Autodesk Inventor part; units mm, degrees
ref_plane "YZ Plane" through (0, 0, 0) normal (1, 0, 0) x (0, 1, 0)
ref_plane "XZ Plane" through (0, 0, 0) normal (0, 1, 0) x (-1, 0, 0)
ref_plane "XY Plane" through (0, 0, 0) normal (0, 0, 1) x (1, 0, 0)
sketch "Szkic1" plane through (0, 0, 0) normal (1, 0, 0) x (0, 1, 0)
  line L0 (-11.2, 0) -> (11.2, 0)
  line L1 (0, -11.2) -> (0, 11.2)
  circle A0 centre (0, 0) radius 8
  dimension "d0" = 16
extrude "Wyciągnięcie proste1" add sketch "Szkic1" along normal blind 212
sketch "Szkic2" plane through (212, 0, 0) normal (1, 0, 0) x (0, 0, -1)
  circle A0 centre (0, 0) radius 8
  line L0 (0, -11.2) -> (0, 11.2)
  line L1 (16, 0) -> (-12, 0)
  circle A1 centre (-4, 0) radius 1
  circle A2 centre (4, 0) radius 1
  point P0 (12, 0)
  dimension "d11" = 10
  dimension "d4" = 16
  dimension "d5" = 2
  dimension "d8" = 8
extrude "Wyciągnięcie proste2" add sketch "Szkic2" along normal blind 7 contours A2 L1 | L1 A2 | A1 L1 | L1 A1
sketch "Szkic3" plane through (0, 0, 0) normal (-1, 0, 0) x (0, 0, 1)
  circle A0 centre (0, 0) radius 8
  line L0 (-11.2, 0) -> (11.2, 0)
  line L1 (0, -11.2) -> (0, 11.2)
  circle A1 centre (-4, 0) radius 1
  circle A2 centre (4, 0) radius 1
  dimension "d19" = 10
  dimension "d15" = 2
  dimension "d16" = 16
  dimension "d22" = 8
extrude "Wyciągnięcie proste3" add sketch "Szkic3" along normal blind 7 contours A2 L0 | L0 A2 | A1 L0 | L0 A1
equation "\"d8\" = 0.5 * d4"
equation "\"d22\" = 0.5 * d16"
properties part number "świetlówka"
Could you check a few things on this model? Use its own coordinates, in mm. Coordinates: 2 decimals unless noted, no trailing zeros. Loops run counter-clockwise (first coordinate to the right, second up) from the corner with the lowest first, then second, coordinate; pieces in that order, holes last. Notation, with made-up numbers: M -37,-27 L -16,-27 A12 ccw -16,-16 Z; hole C 55,-20.75 d11. An arc over 180 degrees is marked long. Put each result on its own line as item: value. Start each with the question number.
(1) Suppose I cut it at B-B on y = -4. Please give me the cut outline in (x, z), then the cut area to 3 significant figures.
(2) I need wall thicknesses on line 1 (X direction, y = 4.75, z = 0); line 2 (Y direction, x = 120, z = 0.25); line 3 (Y direction, x = 32, z = -6.25). Which ranges of each line are inside material? Lowest first, please. Write a range as from..to.
(3) Suppose I cut it at A-A on z = 0. Please give me the cut outline in (x, y), then the cut area to 3 significant figures.
(4) Will these pins go through, and if not, where does the flat tip stop? P1, Ø3, axis at x = 22.5, z = -2, coming from the -Y side; P2, Ø6, axis at x = 184, y = 5.5, coming from the +Z side; P3, Ø4, axis at x = 171.5, z = 5.5, coming from the -Y side.
Solutions:
1. outline: M 0,-6.93 L 212,-6.93 L 212,6.93 L 0,6.93 Z
1. area: 2,940 mm2
2. line 1: x = 0..212
2. line 2: y = -8..8
2. line 3: y = -4.99..4.99
3. outline: M 0,-8 L 212,-8 L 212,8 L 0,8 Z
3. area: 3,390 mm2
4. P1: stops at y = -7.98
4. P2: stops at z = 7.6
4. P3: stops at y = -7.19
